```python
from build123d import *
from build123d.topology import SkipClean

# Parameters (mm, degrees)
SKETCH1_R           = 30
BOSS_EXTRUDE1_DEPTH = 25
FILLET1_R           = 3
SKETCH3_R           = 22.5
CUT_EXTRUDE1_DEPTH  = 20
CHAMFER1_SIZE       = 3
CUT_EXTRUDE2_DEPTH  = 50.244289131
CIRPATTERN1_COUNT   = 5
CIRPATTERN1_ANGLE   = 284
SKETCH4_R           = 12.5
BOSS_EXTRUDE2_DEPTH = 15
SKETCH5_R           = 8.25
CUT_EXTRUDE3_DEPTH  = 47.904157726
SKETCH6_R           = 10
SKETCH6_R_2         = 5
BOSS_EXTRUDE3_DEPTH = 3


with BuildPart() as part:
    # Sketch1 → Boss-Extrude1 (new body)
    with BuildSketch(Plane(origin=(0, 0, 0), x_dir=(0, 0, -1), z_dir=(1, 0, 0))):
        Circle(SKETCH1_R)
    extrude(amount=BOSS_EXTRUDE1_DEPTH)

    # Fillet1
    fillet1_edges = [part.edges().sort_by_distance(p)[0] for p in [
        (0, 0, 30),
        (25, 0, 30),
    ]]
    fillet(fillet1_edges, radius=FILLET1_R)

    # Sketch3 → Cut-Extrude1 (cut)
    with BuildSketch(Plane.ZY):
        Circle(SKETCH3_R)
    extrude(amount=-CUT_EXTRUDE1_DEPTH, mode=Mode.SUBTRACT)

    # Chamfer1
    chamfer1_edges = [part.edges().sort_by_distance(p)[0] for p in [
        (0, 0, -22.5),
    ]]
    chamfer(chamfer1_edges, length=CHAMFER1_SIZE)

    # Sketch2 → Cut-Extrude2 (cut, through all)
    with BuildSketch(Plane.ZY.offset(-25)):
        with BuildLine():
            Line((-6.233158363, 10.835023619), (-11.219685054, 19.503042514))
            ThreePointArc((-11.219685054, 19.503042514), (-15.885142396, 15.934624283), (-19.468053536, 11.280287741))
            Line((-19.468053536, 11.280287741), (-10.815585298, 6.266826523))
            ThreePointArc((-10.815585298, 6.266826523), (-8.825079109, 8.852569046), (-6.233158363, 10.835023619))
        make_face()
    cut_extrude2 = extrude(amount=CUT_EXTRUDE2_DEPTH, mode=Mode.SUBTRACT)

    # CirPattern1: Cut-Extrude2 ×5 about axis
    with SkipClean():  # the faces are left unmerged after this step: merging them gives an invalid solid
        cirpattern1_axis = Axis((0, 0, 0), (1, 0, 0))
        for i in range(1, CIRPATTERN1_COUNT):
            add(cut_extrude2.rotate(cirpattern1_axis, i * CIRPATTERN1_ANGLE / (CIRPATTERN1_COUNT - 1)), mode=Mode.SUBTRACT)
    add(part.part.scale(1), mode=Mode.REPLACE)  # the faces are merged on a copy

    # Sketch4 → Boss-Extrude2 (add)
    with BuildSketch(Plane.ZY.offset(-20)):
        with Locations(Location((0, 0, 0), (0, 0, 195.910901264))):
            Circle(SKETCH4_R)
    extrude(amount=BOSS_EXTRUDE2_DEPTH)

    # Sketch5 → Cut-Extrude3 (cut, through all)
    with BuildSketch(Plane.ZY.offset(-5)):
        Circle(SKETCH5_R)
    extrude(amount=-CUT_EXTRUDE3_DEPTH, mode=Mode.SUBTRACT)

    # Sketch6 → Boss-Extrude3 (add)
    with BuildSketch(Plane.ZY.offset(-5)):
        Circle(SKETCH6_R)
        Circle(SKETCH6_R_2, mode=Mode.SUBTRACT)
    extrude(amount=-BOSS_EXTRUDE3_DEPTH)


solid = part.part
```
Design review of the part built by this model. Coordinates are the model's own, in mm. A direction names the side the tool comes from. Give positions to 0.01 mm unless a question says otherwise; leave off trailing zeros. Write each question's results on one line, items separated by ' | '.
Q1. Wall thickness on L1, parallel to Y at x = 7, z = 0; L2, parallel to Y at x = 15.75, z = 0; L3, parallel to Z at x = 19.75, y = -11: over which ranges is each line inside the solid? List them lowest first.
Reply:
L1: y = -30 to -22.5, -12.5 to -5, 5 to 12.5, 22.5 to 30 | L2: y = -30 to -22.5, -12.5 to -8.25, 8.25 to 12.5, 22.5 to 30 | L3: z = -27.91 to -19.63, -5.94 to 5.94, 19.63 to 27.91
Q2. The part is to be moulded in two halves that separate along Z. For faces 5 (the face through (25, -6, 6)), 6 (the face through (16.38, -3.16, 7.62)), 7 (the face through (12.37, 1.32, 29.97)), say which applies: +Z half, -Z half, draft (parallel to the pull), parting line (faces both ways), or undercut.
Reply:
face 5: draft | face 6: undercut | face 7: parting line
Q3. Machinability: for faces 1 (the face through (8, -4, 4)), 2 (the face through (20, 8, 15)), 3 (the face through (0, -10, -24)), 4 (the face through (22.54, 17.24, 3.38)), which of the approach directions +Z, -Z, +X, -X, +Y, -Y give a long, thin tool a straight path to every point of the face, cutting with its end or side? Answer none if there is none.
Reply:
face 1: +X | face 2: -X | face 3: +Z, -Z, -X, +Y, -Y | face 4: +X, -X
Q4. For pin 1 Ø8 at (x, y) = (12, 21) entering from -Z; pin 2 Ø4 at (x, y) = (11, -15.5) entering from -Z; pin 3 Ø6 at (x, z) = (6, 9.5) entering from -Y, all flat-tipped, find the tip position at first contact; note any pin that passes through.
Reply:
pin 1: stops at z = -24.72 | pin 2: stops at z = -26.79 | pin 3: stops at y = -29.29
Q5. Take a section at A-A, the plane z = 14. Give the number of separate pieces and of enclosed holes in the cut face, plus the area to 3 significant figures.
Reply:
separate pieces: 3 | enclosed holes: 0 | area: 556 mm²
